Here's how the part is built. I have some questions about the finished solid (model axes, mm). A direction names the side the tool comes from. Coordinates: 2 decimals unless noted, no trailing zeros. Order: outer loops, then holes, each group sorted by start corner. A loop starts at its lowest first (then second) coordinate and runs counter-clockwise, first axis right, second up. Notation, with made-up numbers: M -31,69 L -3,69 A15 ccw -3,85 Z; hole C 36,-26 d10. An arc over 180 degrees is marked long. Answer as CSV lines item,"result". Start each with the question number.
```python
from build123d import *

# Parameters (mm, degrees)
SKETCH1_W                       = 40
SKETCH1_H                       = 28
BOSS_EXTRUDE1_DEPTH             = 2
SKETCH2_W                       = 20
SKETCH2_H                       = 4
BOSS_EXTRUDE2_DEPTH             = 20
FILLET1_R                       = 10
F_10_0MM_DOWEL_HOLE1_D          = 13
F_2_0MM_DOWEL_HOLE1_D           = 2
F_2_0MM_DOWEL_HOLE1_CSINK_D     = 2.05
F_2_0MM_DOWEL_HOLE1_CSINK_ANGLE = 90
FILLET2_R                       = 3


with BuildPart() as part:
    # Sketch1 → Boss-Extrude1 (new body)
    with BuildSketch(Plane(origin=(0, 0, 0), x_dir=(0, 1, 0), z_dir=(0, 0, 1))):
        Rectangle(SKETCH1_W, SKETCH1_H)
    extrude(amount=-BOSS_EXTRUDE1_DEPTH)

    # Sketch2 → Boss-Extrude2 (add)
    with BuildSketch(Plane(origin=(0, 0, 0), x_dir=(0, 1, 0), z_dir=(0, 0, 1))):
        with Locations((0, 12)):
            Rectangle(SKETCH2_W, SKETCH2_H)
        with Locations((0, -12)):
            Rectangle(SKETCH2_W, SKETCH2_H)
    extrude(amount=BOSS_EXTRUDE2_DEPTH)

    # Fillet1
    fillet1_edges = [part.edges().sort_by_distance(p)[0] for p in [
        (12, 10, 20),
        (12, -10, 20),
        (-12, 10, 20),
        (-12, -10, 20),
    ]]
    fillet(fillet1_edges, radius=FILLET1_R - 0.0001)  # a hair under: the kernel refuses the full size

    # Ø10.0mm Dowel Hole1 (through all)
    with Locations(Plane.YZ.offset(14)):
        with Locations((0, 10)):
            Hole(F_10_0MM_DOWEL_HOLE1_D / 2)

    # Ø2.0mm Dowel Hole1 (through all)
    with Locations(Plane(origin=(0, 0, 0), x_dir=(0, 1, 0), z_dir=(0, 0, 1))):
        with Locations((15, -7.5), (-15, 7.5), (-15, -7.5), (15, 7.5)):
            CounterSinkHole(F_2_0MM_DOWEL_HOLE1_D / 2, F_2_0MM_DOWEL_HOLE1_CSINK_D / 2, counter_sink_angle=F_2_0MM_DOWEL_HOLE1_CSINK_ANGLE)

    # Fillet2
    fillet2_edges = [part.edges().sort_by_distance(p)[0] for p in [
        (-12, -10, 0),
        (-12, 10, 0),
        (12, -10, 0),
        (12, 10, 0),
        (-14, -20, -1),
        (-14, 20, -1),
        (14, 20, -1),
        (14, -20, -1),
    ]]
    fillet(fillet2_edges, radius=FILLET2_R)


solid = part.part
```
1) Suppose I cut it at D-D on x = -2.75. Please give me the cut outline in (y, z), plus the area to 3 significant figures.
2) Will these pins go through, and if not, where does the flat tip stop? pin 1 Ø4 at (x, z) = (9.5, 16) entering from +Y; pin 2 Ø3 at (x, z) = (-12, 6.5) entering from -Y; pin 3 Ø8 at (x, z) = (7, 16.5) entering from +Y.
3) Suppose I cut it at A-A on y = -15. Please give me the cut outline in (x, z) (3 decimals), plus the area to 3 significant figures.
4) I need wall thicknesses on line 1 (Y direction, x = -7.5, z = -0.95); line 2 (X direction, y = -15, z = -0.7); line 3 (Z direction, x = 11.1, y = 0). Which ranges of each line are inside material? Lowest first, please. Write a range as [from, to].
5) Suppose I cut it at B-B on z = 13.25. Please give me the cut outline in (x, y).
6) Which directions (+Z, -Z, +X, -X, +Y, -Y) give clear straight access to the entire face, cutting with the end or side of a thin tool? Please do faces 1 (the face through (-10, 0, 3)), 2 (the face through (-12, -10, 6)), 3 (the face through (12, 10, 6)).
7) If we mould it in two halves opening along X, with no side actions, what happens to faces 4 (the face through (-12.03, -10.86, 0.9)), 5 (the face through (-7.8, -15.954, -1.026)), 6 (the face through (13.14, -19.1, -1.01))? For each: released by +X, released by -X, zero draft, split by the parting line, or undercut.
8) Suppose I cut it at C-C on z = 17. Please give me the cut outline in (x, y), plus the area to 3 significant figures.
Output:
1,outline,"M -20,-2 L 20,-2 L 20,0 L -20,0 Z"
1,area,"80.0 mm²"
2,pin 1,"y = 9.14"
2,pin 2,"y = -10"
2,pin 3,"y = 9.23"
3,outline,"M -14,-2 L -8.5,-2 L -8.5,-0.025 L -8.525,0 L -14,0 Z; M -6.5,-2 L 6.5,-2 L 6.5,-0.025 L 6.475,0 L -6.475,0 L -6.5,-0.025 Z; M 8.5,-2 L 14,-2 L 14,0 L 8.525,0 L 8.5,-0.025 Z"
3,area,"48.0 mm²"
4,line 1,"[-20, -16], [-14, 14], [16, 20]"
4,line 2,"[-14, -8.5], [-6.5, 6.5], [8.5, 14]"
4,line 3,"[-2, 3.5], [16.5, 20]"
5,outline,"M -14,-9.46 L -10,-9.46 L -10,-5.63 L -14,-5.63 Z; M -14,5.63 L -10,5.63 L -10,9.46 L -14,9.46 Z; M 10,-9.46 L 14,-9.46 L 14,-5.63 L 10,-5.63 Z; M 10,5.63 L 14,5.63 L 14,9.46 L 10,9.46 Z"
6,face 1,"+Z, +Y, -Y"
6,face 2,"+Z, +X, -X, -Y"
6,face 3,"+Z, +X, -X, +Y"
7,face 4,"zero draft"
7,face 5,"undercut"
7,face 6,"released by +X"
8,outline,"M -14,-7.14 L -10,-7.14 L -10,7.14 L -14,7.14 Z; M 10,-7.14 L 14,-7.14 L 14,7.14 L 10,7.14 Z"
8,area,"114 mm²"
